Read the model definition and answer for the solid it produces. Units are mm, in the model's axes. Face numbers are marked on the shaded views. A direction names the side the tool comes from. Round coordinates to 2 decimals unless told otherwise and drop trailing zeros. Order: outer loops, then holes, each group sorted by start corner. A loop starts at its lowest first (then second) coordinate and runs counter-clockwise, first axis right, second up. Notation, with made-up numbers: (7, 32) - (21, 32) arc R12 cw to (21, 54) - close; hole circle Ø8 at (53.5, -17.5). An arc over 180 degrees is marked (long way). Answer as a JSON object with one key per item and string values. Group by question number.
Q1. A cutting plane is placed at C-C on y = 136.5. Determine the outline of the cut face in (x, z), and give its area (3 significant figures).
Q2. Consider line 1 (X direction, y = 156.5, z = 23); line 2 (X direction, y = 6, z = 13.5); line 3 (Y direction, x = -16, z = 38). Determine where each line is inside the solid, lowest interval first.
Q3. A cutting plane is placed at A-A on z = 0. Determine the outline of the cut face in (x, y).
Q4. Given pin 1 Ø11.5 at (y, z) = (160.5, 35.5) entering from -X; pin 2 Ø1.5 at (x, y) = (1, 55) entering from +Z; pin 3 Ø12.5 at (y, z) = (165, 29) entering from +X; pin 4 Ø7.5 at (y, z) = (0, 38.1) entering from +X, each flat-ended and moving along its own axis, determine where each tip first touches the part or whether it passes through.
Q5. The mould has two halves that part along X. Classify the marked faces 1, 2, 3 and 4: pulls with the +X half, pulls with the -X half, needs draft (parallel to the pull), parting line crosses it, or undercut.
Q6. A tool of negligible diameter and unlimited length cuts with its end or side. For the marked faces 5, 6 and 7, from which of +Z, -Z, +X, -X, +Y, -Y can it reach the whole face along a straight path? Write none if from no direction.
Q7. A cutting plane is placed at D-D on z = -9.5. Determine the outline of the cut face in (x, y).
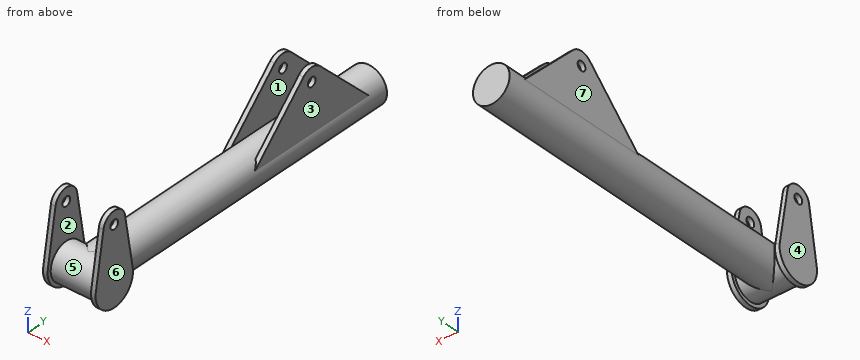
```python
from build123d import *

# Parameters (mm, degrees)
SKETCH1_R           = 12.7
BOSS_EXTRUDE1_DEPTH = 15.0495
BOSS_EXTRUDE2_START = 18.2245
SKETCH1_6_R         = 12.7
SKETCH1_6_R_2       = 3.175
BOSS_EXTRUDE2_DEPTH = 3.175
BOSS_EXTRUDE3_START = 8.382
SKETCH1_8_R         = 3.175
BOSS_EXTRUDE3_DEPTH = 3.175
SKETCH2_R           = 12.7
BOSS_EXTRUDE4_DEPTH = 228.6


with BuildPart() as part:
    # Sketch1 → Boss-Extrude1 (new, symmetric)
    with BuildSketch(Plane.YZ):
        with Locations(Location((0, 0, 0), (0, 0, 90))):
            Circle(SKETCH1_R)
    extrude(amount=BOSS_EXTRUDE1_DEPTH, both=True)

    # Sketch1<6> → Boss-Extrude2 (add)
    # profile 1 of 2: a face of its own
    with BuildSketch(Plane.YZ.offset(BOSS_EXTRUDE2_START)):
        with BuildLine():
            Line((8.765658212, 39.581666667), (15.026842649, 2.54))
            ThreePointArc((15.026842649, 2.54), (0, -15.24), (-15.026842649, 2.54))
            Line((-15.026842649, 2.54), (-8.765658212, 39.581666667))
            ThreePointArc((-8.765658212, 39.581666667), (0, 46.99), (8.765658212, 39.581666667))
        make_face()
        with Locations(Location((0, 0, 0), (0, 0, 90))):
            Circle(SKETCH1_6_R, mode=Mode.SUBTRACT)
        with Locations(Location((0, 38.1, 0), (0, 0, 270))):
            Circle(SKETCH1_6_R_2, mode=Mode.SUBTRACT)
    # profile 2 of 2: a face of its own
    with BuildSketch(Plane.YZ.offset(BOSS_EXTRUDE2_START)):
        with Locations(Location((0, 0, 0), (0, 0, 90))):
            Circle(SKETCH1_6_R)
    extrude(amount=-BOSS_EXTRUDE2_DEPTH)



with BuildPart() as body_2:
    # Sketch1<8> → Boss-Extrude3 (new body)
    with BuildSketch(Plane.YZ.offset(BOSS_EXTRUDE3_START)):
        with BuildLine():
            Line((161.946207909, 44.835192091), (117.111015818, 0))
            Line((117.111015818, 0), (220.251784182, 0))
            Line((220.251784182, 0), (175.416592091, 44.835192091))
            ThreePointArc((175.416592091, 44.835192091), (168.6814, 47.625), (161.946207909, 44.835192091))
        make_face()
        with Locations(Location((168.6814, 38.1, 0), (0, 0, 270))):
            Circle(SKETCH1_8_R, mode=Mode.SUBTRACT)
    extrude(amount=BOSS_EXTRUDE3_DEPTH)


with BuildPart() as part_1:
    add(part.part)

    add(body_2.part)  # Boss-Extrude4 merges body 2
    # Sketch2 → Boss-Extrude4 (add)
    with BuildSketch(Plane(origin=(0, 0, 0), x_dir=(-1, 0, 0), z_dir=(0, 1, 0))):
        with Locations(Location((0, 0, 0), (0, 0, 90))):
            Circle(SKETCH2_R)
    extrude(amount=BOSS_EXTRUDE4_DEPTH)

    # Mirror1: part across plane


with BuildPart() as part_2:
    add(part_1.part)
    add(part_1.part.mirror(Plane(origin=(0, 0, 0), x_dir=(0, 0, 1), z_dir=(1, 0, 0))))


solid = part_2.part
```
Result set:
{
 "1": {"outline": "(-11.56, 5.27) arc R12.7 ccw (long way) to (11.56, 5.27) - (11.56, 19.39) - (8.38, 19.39) - (8.38, 9.54) arc R12.7 ccw to (-8.38, 9.54) - (-8.38, 19.39) - (-11.56, 19.39) - close", "area": "581 mm²"},
 "2": {"line 1": "x = -11.56 to -8.38, 8.38 to 11.56", "line 2": "x = -18.22 to -15.05, 15.05 to 18.22", "line 3": "y = -9.03 to -3.17, 3.17 to 9.03"},
 "3": {"outline": "(-18.22, -15.24) - (-15.05, -15.24) - (-15.05, -12.7) - (15.05, -12.7) - (15.05, -15.24) - (18.22, -15.24) - (18.22, 15.24) - (15.05, 15.24) - (15.05, 12.7) - (12.7, 12.7) - (12.7, 228.6) - (-12.7, 228.6) - (-12.7, 12.7) - (-15.05, 12.7) - (-15.05, 15.24) - (-18.22, 15.24) - close"},
 "4": {"pin 1": "stops at x = -11.56", "pin 2": "stops at z = 12.7", "pin 3": "stops at x = 11.56", "pin 4": "stops at x = 18.22"},
 "5": {"face 1": "undercut", "face 2": "undercut", "face 3": "pulls with the +X half", "face 4": "pulls with the -X half"},
 "6": {"face 5": "none", "face 6": "+Z, -Z, +X, +Y, -Y", "face 7": "+Z, -X, +Y"},
 "7": {"outline": "(-18.22, -11.92) - (-15.05, -11.92) - (-15.05, -8.43) - (15.05, -8.43) - (15.05, -11.92) - (18.22, -11.92) - (18.22, 11.92) - (15.05, 11.92) - (15.05, 8.43) - (8.43, 8.43) - (8.43, 228.6) - (-8.43, 228.6) - (-8.43, 8.43) - (-15.05, 8.43) - (-15.05, 11.92) - (-18.22, 11.92) - close"}
}
